```python
from build123d import *

# Parameters (mm, degrees)
BOSS_EXTRUDE1_REACH     = 84.183
CUT_EXTRUDE1_DEPTH      = 91.676766104
CUT_EXTRUDE1_DEPTH_BACK = 91.676766104
GUDGEON_HOLE_R          = 11
CUT_EXTRUDE2_DEPTH      = 114.265175749
RING_CS_W               = 2
RING_CS_H               = 1
BOSS_EXTRUDE2_DEPTH     = 3
FILLET1_R               = 3


with BuildPart() as part:
    # Piston CS → Revolve1 (revolve)
    with BuildSketch(Plane.XY, mode=Mode.PRIVATE) as revolve1_sk:
        Polygon((0, 0), (0, -5), (2.220419784, -5), (37, -25.08), (37, -35.08), (42, -35.08), (42, -52), (45, -52), (45, -5), (44, -5), (35.339745962, 0), align=None)
    revolve(revolve1_sk.sketch.rotate(Axis((0, 0, 0), (0, -1, 0)), 90), axis=Axis((0, 0, 0), (0, -1, 0)))

    # Sketch5 → Boss-Extrude1 (add, up to next)
    with BuildSketch(Plane.XZ.offset(52), mode=Mode.PRIVATE) as boss_extrude1_sk1:
        with BuildLine():
            Line((-24.103941586, -38), (-24.103941586, -15))
            Line((-24.103941586, -15), (-14.103941586, -15))
            Line((-14.103941586, -15), (-14.103941586, 15))
            Line((-14.103941586, 15), (-24.103941586, 15))
            Line((-24.103941586, 15), (-24.103941586, 38))
            ThreePointArc((-24.103941586, 38), (-45, 0), (-24.103941586, -38))
        make_face()
    boss_extrude1_tool1 = extrude(boss_extrude1_sk1.sketch, amount=-BOSS_EXTRUDE1_REACH, mode=Mode.PRIVATE) - part.part
    # Sketch5 → Boss-Extrude1 (add, up to next)
    with BuildSketch(Plane.XZ.offset(52), mode=Mode.PRIVATE) as boss_extrude1_sk2:
        with BuildLine():
            Line((24.103941586, 38), (24.103941586, 15))
            Line((24.103941586, 15), (14.103941586, 15))
            Line((14.103941586, 15), (14.103941586, -15))
            Line((14.103941586, -15), (24.103941586, -15))
            Line((24.103941586, -15), (24.103941586, -38))
            ThreePointArc((24.103941586, -38), (45, 0), (24.103941586, 38))
        make_face()
    boss_extrude1_tool2 = extrude(boss_extrude1_sk2.sketch, amount=-BOSS_EXTRUDE1_REACH, mode=Mode.PRIVATE) - part.part
    add(boss_extrude1_tool1.solids().sort_by_distance((-29.792455, -52, 0))[0])
    add(boss_extrude1_tool2.solids().sort_by_distance((29.792455, -52, 0))[0])

    # Gudgeon Hole → Cut-Extrude1 (cut, two sides: drawn at the far end of the back side and taken through both)
    with BuildSketch(Plane(origin=(-14.103941586, 0, 0), x_dir=(0, 0, -1), z_dir=(1, 0, 0)).offset(-CUT_EXTRUDE1_DEPTH_BACK)):
        with Locations((0, -26)):
            Circle(GUDGEON_HOLE_R)
    extrude(amount=CUT_EXTRUDE1_DEPTH + CUT_EXTRUDE1_DEPTH_BACK, mode=Mode.SUBTRACT)

    # Gudgeon Hole Cutouts → Cut-Extrude2 (cut, through all)
    with BuildSketch(Plane.XY.offset(45)):
        with BuildLine():
            Line((-42, -15), (-45, -15))
            add(Edge.make_bspline(
                [(-45, -15), (-42.311111111, -26), (-45, -37)],
                knots=[0, 0, 0, 1, 1, 1], degree=2, weights=[0.034, 0.045, 0.056]))
            Line((-45, -37), (-42, -37))
            Line((-42, -37), (-42, -15))
        make_face()
        with BuildLine():
            Line((42, -37), (45, -37))
            add(Edge.make_bspline(
                [(45, -37), (42.311111111, -26), (45, -15)],
                knots=[0, 0, 0, 1, 1, 1], degree=2, weights=[0.034, 0.045, 0.056]))
            Line((45, -15), (42, -15))
            Line((42, -15), (42, -37))
        make_face()
    extrude(amount=-CUT_EXTRUDE2_DEPTH, mode=Mode.SUBTRACT)

    # Ring CS → Cut-Revolve1 (revolve, cut)
    with BuildSketch(Plane.XY, mode=Mode.PRIVATE) as cut_revolve1_sk:
        with Locations((44, -6.5)):
            Rectangle(RING_CS_W, RING_CS_H)
        with Locations((44, -9.5)):
            Rectangle(RING_CS_W, RING_CS_H)
        with Locations((44, -12.5)):
            Rectangle(RING_CS_W, RING_CS_H)
    revolve(cut_revolve1_sk.sketch.rotate(Axis((0, 0, 0), (0, -1, 0)), 90), axis=Axis((0, 0, 0), (0, -1, 0)), mode=Mode.SUBTRACT)

    # Sketch9 → Boss-Extrude2 (add)
    with BuildSketch(Plane.XZ.offset(52)):
        with BuildLine():
            Line((-1.832014269, 41.960025306), (-1.962872431, 44.957169971))
            ThreePointArc((-1.962872431, 44.957169971), (0, 45), (1.962872431, 44.957169971))
            Line((1.962872431, 44.957169971), (1.832014269, 41.960025306))
            ThreePointArc((1.832014269, 41.960025306), (0, 42), (-1.832014269, 41.960025306))
        make_face()
        with BuildLine():
            Line((1.832014269, -41.960025306), (1.962872431, -44.957169971))
            ThreePointArc((1.962872431, -44.957169971), (0, -45), (-1.962872431, -44.957169971))
            Line((-1.962872431, -44.957169971), (-1.832014269, -41.960025306))
            ThreePointArc((-1.832014269, -41.960025306), (0, -42), (1.832014269, -41.960025306))
        make_face()
    extrude(amount=BOSS_EXTRUDE2_DEPTH)

    # Fillet1
    # the kernel refuses this fillet: 3 mm, written as the material it adds along each edge
    with BuildSketch(Plane(origin=(-1.504868864, -52, 34.467163645), x_dir=(-0.999048221581858, 0, -0.043619387365329124), z_dir=(-0.043619387365329124, 0, 0.9990482215818581))) as fillet1_piece_1_section:
        with BuildLine():
            CenterArc((FILLET1_R, FILLET1_R), FILLET1_R, 180, 90)
            Line((0, FILLET1_R), (0, 0))
            Line((0, 0), (FILLET1_R, 0))
        make_face()
    fillet1_piece_1 = extrude(amount=18, mode=Mode.PRIVATE)
    fillet1_piece_1 = fillet1_piece_1 & Plane(origin=(0, -52.679071729, 0), x_dir=(0, 0, 1), z_dir=(0, 1, 0)) * Cylinder(45, 49, mode=Mode.PRIVATE)
    fillet1_piece_1 = fillet1_piece_1 - Plane(origin=(0, -52.679071729, 0), x_dir=(0, 0, 1), z_dir=(0, -1, 0)) * Cylinder(42, 49, mode=Mode.PRIVATE)
    add(fillet1_piece_1)
    with BuildSketch(Plane(origin=(2.290017837, -52, 52.450031633), x_dir=(0.9990482215818575, 0, -0.04361938736534308), z_dir=(-0.04361938736534308, 0, -0.9990482215818575))) as fillet1_piece_2_section:
        with BuildLine():
            CenterArc((FILLET1_R, FILLET1_R), FILLET1_R, 180, 90)
            Line((0, FILLET1_R), (0, 0))
            Line((0, 0), (FILLET1_R, 0))
        make_face()
    fillet1_piece_2 = extrude(amount=18, mode=Mode.PRIVATE)
    fillet1_piece_2 = fillet1_piece_2 - Plane(origin=(0, -52.679065019, 0), x_dir=(0, 0, 1), z_dir=(0, -1, 0)) * Cylinder(42, 49, mode=Mode.PRIVATE)
    fillet1_piece_2 = fillet1_piece_2 & Plane(origin=(0, -52.679065019, 0), x_dir=(0, 0, 1), z_dir=(0, 1, 0)) * Cylinder(45, 49, mode=Mode.PRIVATE)
    add(fillet1_piece_2)
    with BuildSketch(Plane(origin=(1.504868864, -52, -34.467163645), x_dir=(0.9990482215818575, 0, 0.04361938736534308), z_dir=(0.04361938736534308, 0, -0.9990482215818575))) as fillet1_piece_3_section:
        with BuildLine():
            CenterArc((FILLET1_R, FILLET1_R), FILLET1_R, 180, 90)
            Line((0, FILLET1_R), (0, 0))
            Line((0, 0), (FILLET1_R, 0))
        make_face()
    fillet1_piece_3 = extrude(amount=18, mode=Mode.PRIVATE)
    fillet1_piece_3 = fillet1_piece_3 - Plane(origin=(0, -52.679069886, 0), x_dir=(0, 0, 1), z_dir=(0, -1, 0)) * Cylinder(42, 49, mode=Mode.PRIVATE)
    fillet1_piece_3 = fillet1_piece_3 & Plane(origin=(0, -52.679069886, 0), x_dir=(0, 0, 1), z_dir=(0, 1, 0)) * Cylinder(45, 49, mode=Mode.PRIVATE)
    add(fillet1_piece_3)
    with BuildSketch(Plane(origin=(-2.290017837, -52, -52.450031633), x_dir=(-0.999048221581858, 0, 0.04361938736532913), z_dir=(0.043619387365329124, 0, 0.9990482215818581))) as fillet1_piece_4_section:
        with BuildLine():
            CenterArc((FILLET1_R, FILLET1_R), FILLET1_R, 180, 90)
            Line((0, FILLET1_R), (0, 0))
            Line((0, 0), (FILLET1_R, 0))
        make_face()
    fillet1_piece_4 = extrude(amount=18, mode=Mode.PRIVATE)
    fillet1_piece_4 = fillet1_piece_4 - Plane(origin=(0, -52.679069383, 0), x_dir=(0, 0, 1), z_dir=(0, -1, 0)) * Cylinder(42, 49, mode=Mode.PRIVATE)
    fillet1_piece_4 = fillet1_piece_4 & Plane(origin=(0, -52.679069383, 0), x_dir=(0, 0, 1), z_dir=(0, 1, 0)) * Cylinder(45, 49, mode=Mode.PRIVATE)
    add(fillet1_piece_4)


solid = part.part
```
Input: part model. Units: mm. Frame: model coordinates. A direction names the side the tool comes from. Coordinates: 2 decimals unless noted, no trailing zeros. Loops run counter-clockwise (first coordinate to the right, second up) from the corner with the lowest first, then second, coordinate; pieces in that order, holes last. Notation, with made-up numbers: M 83.25,-19.5 L 138.25,-19.5 A28 cw 138.25,1.5 Z; hole C 47.5,46.25 d1. An arc over 180 degrees is marked long. Use a Markdown table: item, result. Add a question column.
1) Line query: L1, parallel to Z at x = 1.5, y = -43.5 (3 decimals); L2, parallel to Y at x = -26, z = 0; L3, parallel to Y at x = -36, z = -25.5. Output: solid intervals per line, ascending. Write a range as from..to.
2) Draft query along X for faces 4 (the flat face through (42, -26, 12)), 5 (the cylindrical face through (27.86, -36.74, 2.38)), 6 (the flat face through (-14.104, -37, -4)). Return one class per face: +X half, -X half, draft (parallel to the pull), parting line (faces both ways), or undercut.
3) Pin query (flat end, axial travel): P1, Ø1.5, axis at x = 43.5, z = 7, coming from the +Y side; P2, Ø8, axis at x = -20.5, y = -42.5, coming from the -Z side; P3, Ø24, axis at y = -38.5, z = -2.5, coming from the -X side; P4, Ø5, axis at x = 1, z = -1, coming from the -Y side. Return the tip coordinate at first contact, or that it passes through.
4) Section A-A, the plane y = -32. Return the cut outline in (x, z).
5) Section B-B, the plane z = 8. Give the number of separate pieces and of enclosed holes in the cut face, plus the area to 3 significant figures.
6) Set-up query: faces 1 (the flat face through (36.5, -7, -23.1)), 2 (the cylindrical face through (2.751, -52.902, 43.389)), 3 (the cylindrical face through (0, -30, 37)). Return all of +Z, -Z, +X, -X, +Y, -Y with unobstructed straight access to the full face (end or side cutting, diameter ignored); none if empty.
Answer below:
| question | item | result |
|---|---|---|
| 1 | L1 | -44.975..-41.973, 41.973..44.975 |
| 1 | L2 | -52..-37, -15..0 |
| 1 | L3 | -52..-13, -12..-10, -9..-7, -6..-5 |
| 2 | face 4 | +X half |
| 2 | face 5 | draft |
| 2 | face 6 | undercut |
| 3 | P1 | y = -4.6 |
| 3 | P2 | z = -41.87 |
| 3 | P3 | x = -45 |
| 3 | P4 | y = -5.98 |
| 4 | outline | M -42,-16.16 A45 ccw 42,-16.16 L 42,-9.22 L 14.1,-9.22 L 14.1,-15 L 24.1,-15 L 24.1,-28.07 A37 cw -24.1,-28.07 L -24.1,-15 L -14.1,-15 L -14.1,-9.22 L -42,-9.22 Z; M -42,9.22 L -14.1,9.22 L -14.1,15 L -24.1,15 L -24.1,28.07 A37 cw 24.1,28.07 L 24.1,15 L 14.1,15 L 14.1,9.22 L 42,9.22 L 42,16.16 A45 ccw -42,16.16 Z |
| 5 | separate pieces | 3 |
| 5 | enclosed holes | 0 |
| 5 | area | 2,420 mm2 |
| 6 | face 1 | none |
| 6 | face 2 | +X, -Y |
| 6 | face 3 | -Y |
